Read the model definition and answer for the solid it produces. Units are mm, in the model's axes. Coordinates: 2 decimals unless noted, no trailing zeros. Order: outer loops, then holes, each group sorted by start corner. A loop starts at its lowest first (then second) coordinate and runs counter-clockwise, first axis right, second up. Notation, with made-up numbers: (-17.75, 50.25) - (-11.75, 50.25) arc R18 ccw to (-11.75, 67.25) - close; hole circle Ø6 at (-13, -6.5). An arc over 180 degrees is marked (long way). Write item = value, one per line.
from build123d import *

# Parameters (mm, degrees)
SKETCH1_R           = 4.5
BOSS_EXTRUDE1_DEPTH = 4.5


with BuildPart() as part:
    # Sketch1 → Boss-Extrude1 (new body, symmetric)
    with BuildSketch(Plane(origin=(0, 0, 0), x_dir=(1, 0, 0), z_dir=(0, 1, 0))):
        Polygon((8.660254038, 0), (4.330127019, 7.5), (-4.330127019, 7.5), (-8.660254038, 0), (-4.330127019, -7.5), (4.330127019, -7.5), align=None)
        with Locations(Location((0, 0, 0), (0, 0, 270))):  # turned: the seam where the file's is
            Circle(SKETCH1_R, mode=Mode.SUBTRACT)
    extrude(amount=BOSS_EXTRUDE1_DEPTH, both=True)

    # Sketch3 → Cut-Revolve2 (revolve, cut)
    with BuildSketch(Plane(origin=(0, 0, 0), x_dir=(0, 0, -1), z_dir=(1, 0, 0)), mode=Mode.PRIVATE) as cut_revolve2_sk:
        Polygon((4.215565438, 6.358242553), (9.417491766, 3.354908986), (9.417491766, 6.358242553), align=None)
        Polygon((9.417491766, -6.358242553), (4.215565438, -6.358242553), (9.417491766, -3.354908986), align=None)
    revolve(cut_revolve2_sk.sketch.rotate(Axis((0, 0, 0), (0, 1, 0)), 180), axis=Axis((0, 0, 0), (0, 1, 0)), mode=Mode.SUBTRACT)  # turned: the seam where the file's is

    # Sketch2 → Cut-Revolve1 (revolve, cut)
    with BuildSketch(Plane.XY, mode=Mode.PRIVATE) as cut_revolve1_sk:
        Polygon((4.548999988, 6.358242553), (10.760780108, 2.771869628), (10.760780108, 6.358242553), align=None)
        Polygon((10.760780108, -6.358242553), (4.548999988, -6.358242553), (10.760780108, -2.771869628), align=None)
    revolve(cut_revolve1_sk.sketch.rotate(Axis((0, 0, 0), (0, 1, 0)), 270), axis=Axis((0, 0, 0), (0, 1, 0)), mode=Mode.SUBTRACT)  # turned: the seam where the file's is


solid = part.part
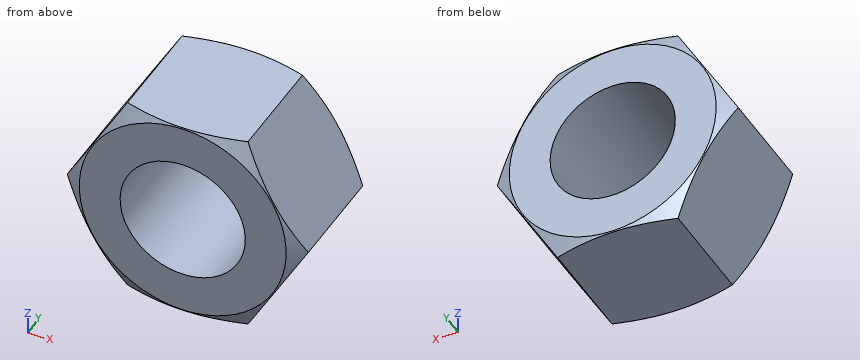
1) The part is cut by section B-B (y = 0.5). Determine the outline of the cut face in (x, z).
Returned:
outline = (-8.66, 0) - (-4.33, -7.5) - (4.33, -7.5) - (8.66, 0) - (4.33, 7.5) - (-4.33, 7.5) - close; hole circle Ø9 at (0, 0)
2) The part is cut by section A-A (x = 0). Determine the outline of the cut face in (y, z).
Returned:
outline = (-4.5, -7.43) - (-4.46, -7.5) - (4.46, -7.5) - (4.5, -7.43) - (4.5, -4.5) - (-4.5, -4.5) - close; (-4.5, 4.5) - (4.5, 4.5) - (4.5, 7.43) - (4.46, 7.5) - (-4.46, 7.5) - (-4.5, 7.43) - close
3) Straight lines are drawn through the part: line 1 along Y through (x, z) = (7.5, 0); line 2 along Z through (x, y) = (-2.25, -3.5); line 3 along X through (y, z) = (2.75, 2). For each, find the intervals that lie inside material, in ascending order. Write a range as from..to.
Returned:
line_1 = -4.46..4.46
line_2 = -7.5..-3.9, 3.9..7.5
line_3 = -7.51..-4.03, 4.03..7.51
4) Flat-ended cylindrical pins translate along their axes: pin 1 Ø5.5 at (x, z) = (0, 0) entering from +Y; pin 2 Ø2 at (y, z) = (-1.5, -4.5) entering from -X. Find the tip coordinate at first contact, or state that the pin passes through.
Returned:
pin_1 = through
pin_2 = -6.64
